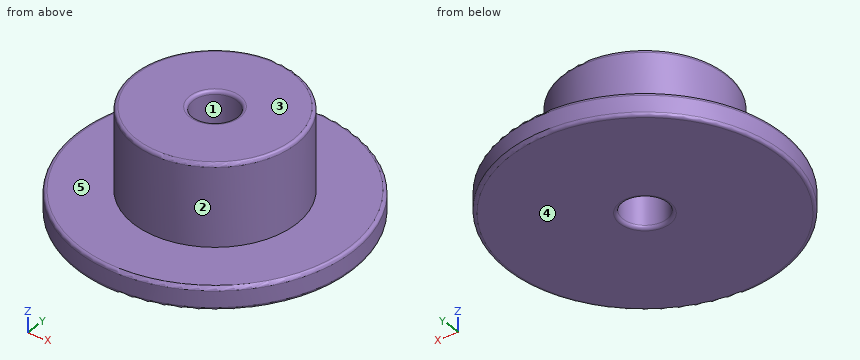
from build123d import *

# Parameters (mm, degrees)
F0_R     = 42.5
F1_DEPTH = 7
F2_R     = 25
F3_DEPTH = 25
F4_R     = 6.75
F5_DEPTH = 32.001
F6_R     = 1


with BuildPart() as f1:
    # F0 (on Top) → F1 (new body)
    with BuildSketch(Plane.XY):
        Circle(F0_R)
    extrude(amount=F1_DEPTH)

    # F2 (on face) → F3 (join)
    with BuildSketch(Plane.XY.offset(7)):
        Circle(F2_R)
    extrude(amount=F3_DEPTH)

    # F4 (on face) → F5 (cut, through all)
    with BuildSketch(Plane.XY.offset(32)):
        Circle(F4_R)
    extrude(amount=-F5_DEPTH, mode=Mode.SUBTRACT)

    # F6
    f6_edges = [f1.edges().sort_by_distance(p)[0] for p in [
        (-6.75, 0, 32),
        (-6.75, 0, 0),
        (-42.5, 0, 0),
        (-42.5, 0, 7),
        (-25, 0, 32),
    ]]
    fillet(f6_edges, radius=F6_R)


solid = f1.part
The listing builds one solid part. Answer for the finished solid, in the listing's coordinates (mm). Face numbers are marked on the shaded views. A direction names the side the tool comes from. Give positions to 0.01 mm unless a question says otherwise; leave off trailing zeros. Loops run counter-clockwise (first coordinate to the right, second up) from the corner with the lowest first, then second, coordinate; pieces in that order, holes last.
Item 1: Find the intervals of material crossed by line 1 along Y through (x, z) = (0, 23); line 2 along X through (y, z) = (0.5, 13) (3 decimals); line 3 along Z through (x, y) = (-3.5, 35.5), in increasing order.
Derived:
line 1: y = -25 to -6.75, 6.75 to 25
line 2: x = -24.995 to -6.731, 6.731 to 24.995
line 3: z = 0 to 7
Item 2: Each of these flat-tipped pins is pushed along its axis until it touches: pin 1 Ø12 at (x, z) = (-26, 23) entering from +Y; pin 2 Ø4 at (x, y) = (-31.5, 13.5) entering from +Z; pin 3 Ø4 at (x, z) = (14, 8.5) entering from +Y; pin 4 Ø11 at (x, y) = (0, 0) entering from +Z. Where does it stop, or does it pass through?
Derived:
pin 1: stops at y = 15
pin 2: stops at z = 7
pin 3: stops at y = 40.13
pin 4: passes through
Item 3: A tool of negligible diameter and unlimited length cuts with its end or side. For the marked faces 4 and 5, from which of +Z, -Z, +X, -X, +Y, -Y can it reach the whole face along a straight path? Write none if from no direction.
Derived:
face 4: -Z, +X, -X, +Y, -Y
face 5: +Z
Item 4: A cutting plane is placed at C-C (z = 20.5). Give the vertices of the cut face in (x, y).
Derived:
outline: circle Ø50 at (0, 0); hole circle Ø13.5 at (0, 0)
Item 5: A cutting plane is placed at A-A (y = 0). Give the vertices of the cut face in (x, z).
Derived:
outline: (-42.5, 1) arc R1 ccw to (-41.5, 0) - (-7.75, 0) arc R1 ccw to (-6.75, 1) - (-6.75, 31) arc R1 ccw to (-7.75, 32) - (-24, 32) arc R1 ccw to (-25, 31) - (-25, 7) - (-41.5, 7) arc R1 ccw to (-42.5, 6) - close; (6.75, 1) arc R1 ccw to (7.75, 0) - (41.5, 0) arc R1 ccw to (42.5, 1) - (42.5, 6) arc R1 ccw to (41.5, 7) - (25, 7) - (25, 31) arc R1 ccw to (24, 32) - (7.75, 32) arc R1 ccw to (6.75, 31) - close
Item 6: Determine the mould class of the marked faces 1, 2 and 3 for opening direction Y: +Y half, -Y half, draft (parallel to the pull), parting line (faces both ways), or undercut.
Derived:
face 1: undercut
face 2: parting line
face 3: draft
Item 7: A cutting plane is placed at D-D (z = 3). Give the vertices of the cut face in (x, y).
Derived:
outline: circle Ø85 at (0, 0); hole circle Ø13.5 at (0, 0)
